Could you check a few things on this drawing? It's one solid part, dimensions in mm from its lowest x, y, z. Round coordinates to 2 decimals unless told otherwise and drop trailing zeros. Loops run counter-clockwise (first coordinate to the right, second up) from the corner with the lowest first, then second, coordinate; pieces in that order, holes last. Notation, with made-up numbers: M 6,-17 L 38,-17 A16 cw 38,-3 Z; hole C 34,-31.5 d3. An arc over 180 degrees is marked long. Answer as a JSON object with one key per item and string values.
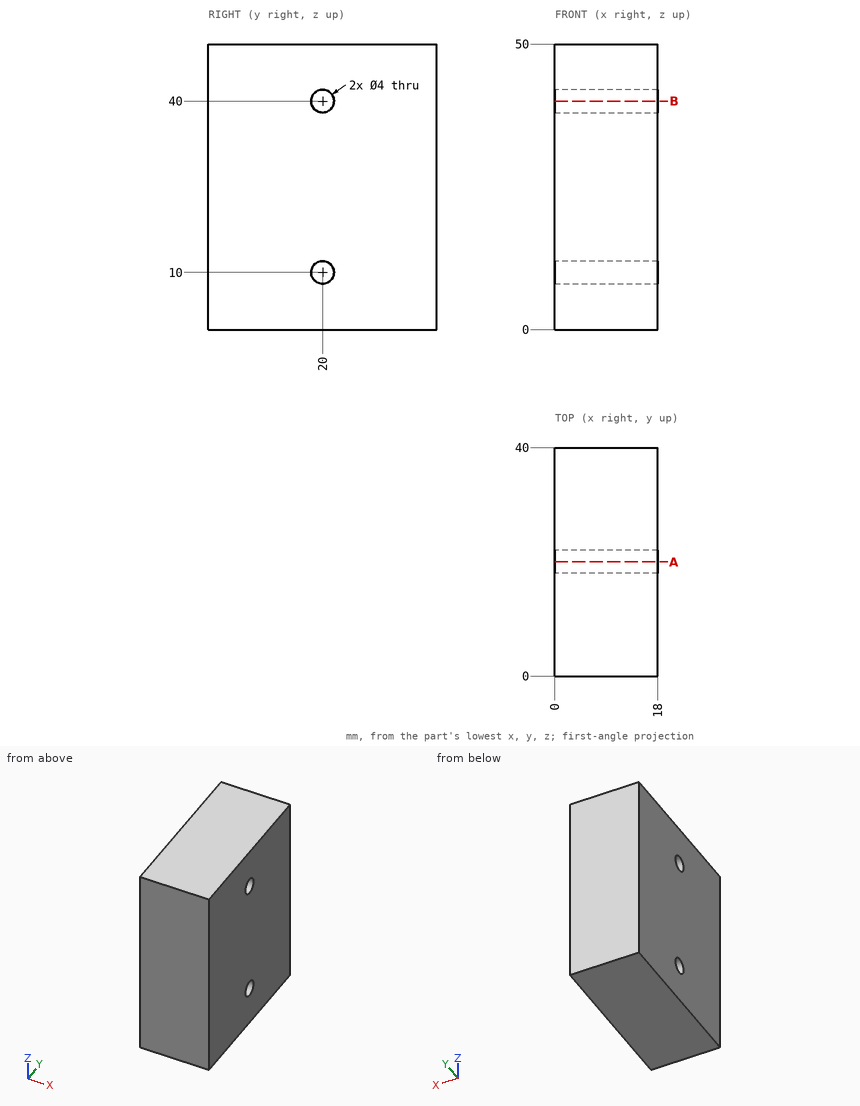
Item 1: Please list where these lines run through material, in increasing order: probe 1 along Z at (x, y) = (5.25, 20); probe 2 along Y at (x, z) = (11.25, 40); probe 3 along Y at (x, z) = (14, 41). Write a range as from..to.
Resolved:
{"probe 1": "0..8, 12..38, 42..50", "probe 2": "0..18, 22..40", "probe 3": "0..18.27, 21.73..40"}
Item 2: I want a section at B-B, the plane z = 40. Please give me the cut outline in (x, y).
Resolved:
{"outline": "M 0,0 L 18,0 L 18,18 L 0,18 Z; M 0,22 L 18,22 L 18,40 L 0,40 Z"}
Item 3: I want a section at A-A, the plane y = 20. Please give me the cut outline in (x, z).
Resolved:
{"outline": "M 0,0 L 18,0 L 18,8 L 0,8 Z; M 0,12 L 18,12 L 18,38 L 0,38 Z; M 0,42 L 18,42 L 18,50 L 0,50 Z"}
